Design review of the part built by this model. Coordinates are the model's own, in mm. Give positions to 0.01 mm unless a question says otherwise; leave off trailing zeros. Loops run counter-clockwise (first coordinate to the right, second up) from the corner with the lowest first, then second, coordinate; pieces in that order, holes last. Notation, with made-up numbers: (79.25, 87) -> (117.25, 87) arc R26 ccw to (117.25, 102) -> close; hole circle Ø11 at (-30, -34). An arc over 180 degrees is marked (long way). Answer in a Markdown table with one row per item. Add a question column.
(1) Consider section C-C on x = 26. Write out the cut boundary in (y, z), then the cut area to 3 significant figures.
(2) Consider section D-D on z = 1.1. Write out the cut boundary in (x, y) (1 decimal), then the cut area to 3 significant figures.
(3) Consider section B-B on x = 12. Write out the cut boundary in (y, z), then the cut area to 3 significant figures.
(4) For line 1 (Y direction, x = 23.5, z = 0.3); line 2 (X direction, y = 17, z = 1.45); line 3 (Y direction, x = 15, z = 0.15), list the stretches that pass through material, from the lowest coordinate up.
(5) Consider section A-A on y = 16. Write out the cut boundary in (x, z).
(6) For pin 1 (0.9 mm diameter, centred on y = 27.5, z = 0.5, fed in from -X); pin 2 (0.5 mm diameter, centred on x = 46, z = 1, fed in from +Y); pin 3 (0.5 mm diameter, centred on y = 36.5, z = 1, fed in from -X) (3 decimals), all flat-tipped, find the tip position at first contact; note any pin that passes through.
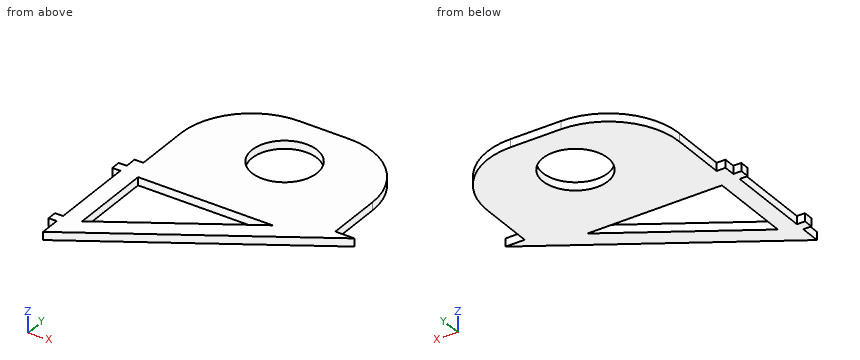
from build123d import *

# Parameters (mm, degrees)
SKETCH1_R           = 7
BOSS_EXTRUDE1_DEPTH = 1.7272
FILLET7_R           = 15.24


with BuildPart() as part:
    # Sketch1 → Boss-Extrude1 (new body)
    with BuildSketch(Plane.XY):
        Polygon((0, 0), (47.288728977, 29.21), (43.18, 29.21), (43.18, 56.3372), (1.905, 56.3372), (1.905, 29.21), (0, 29.21), (0, 26.7208), (-1.7272, 26.7208), (-1.7272, 24.6888), (0, 24.6888), (0, 6.4008), (-1.7272, 6.4008), (-1.7272, 4.3688), (0, 4.3688), align=None)
        with Locations((22.5425, 43.6372)):
            Circle(SKETCH1_R, mode=Mode.SUBTRACT)
        Polygon((3.81, 24.6888), (32.719325319, 24.6888), (3.81, 6.831661294), align=None, mode=Mode.SUBTRACT)
    extrude(amount=BOSS_EXTRUDE1_DEPTH)

    # Fillet7
    fillet7_edges = [part.edges().sort_by_distance(p)[0] for p in [
        (1.905, 56.3372, 0.8636),
        (43.18, 56.3372, 0.8636),
    ]]
    fillet(fillet7_edges, radius=FILLET7_R)


solid = part.part
Values follow:
| question | item | result |
|---|---|---|
| 1 | outline | (16.06, 0) -> (20.54, 0) -> (20.54, 1.73) -> (16.06, 1.73) -> close; (24.69, 0) -> (37.55, 0) -> (37.55, 1.73) -> (24.69, 1.73) -> close; (49.72, 0) -> (56.34, 0) -> (56.34, 1.73) -> (49.72, 1.73) -> close |
| 1 | area | 41.4 mm2 |
| 2 | outline | (-1.7, 4.4) -> (0, 4.4) -> (0, 0) -> (47.3, 29.2) -> (43.2, 29.2) -> (43.2, 41.1) arc R15.2 ccw to (27.9, 56.3) -> (17.1, 56.3) arc R15.2 ccw to (1.9, 41.1) -> (1.9, 29.2) -> (0, 29.2) -> (0, 26.7) -> (-1.7, 26.7) -> (-1.7, 24.7) -> (0, 24.7) -> (0, 6.4) -> (-1.7, 6.4) -> close; hole (3.8, 6.8) -> (32.7, 24.7) -> (3.8, 24.7) -> close; hole circle Ø14 at (22.5, 43.6) |
| 2 | area | 1,310 mm2 |
| 3 | outline | (7.41, 0) -> (11.89, 0) -> (11.89, 1.73) -> (7.41, 1.73) -> close; (24.69, 0) -> (55.44, 0) -> (55.44, 1.73) -> (24.69, 1.73) -> close |
| 3 | area | 60.9 mm2 |
| 4 | line 1 | 14.52 to 18.99, 24.69 to 36.7, 50.57 to 56.34 |
| 4 | line 2 | 0 to 3.81, 20.27 to 27.52 |
| 4 | line 3 | 9.27 to 13.74, 24.69 to 56.19 |
| 5 | outline | (0, 0) -> (3.81, 0) -> (3.81, 1.73) -> (0, 1.73) -> close; (18.65, 0) -> (25.9, 0) -> (25.9, 1.73) -> (18.65, 1.73) -> close |
| 6 | pin 1 | x = 0 |
| 6 | pin 2 | y = 29.21 |
| 6 | pin 3 | x = 1.905 |
